```python
from build123d import *

# Parameters (mm, degrees)
F1_R     = 3.429
F2_DEPTH = 2.54
F3_DEPTH = 25.4


# Not quite as in the source:
# - a feature names something its author has since deleted; it is built from what else it names


with BuildPart() as f2:
    # F1 (on offset) → F2 (new body)
    with BuildSketch(Plane.XZ.offset(25.4)):
        with BuildLine():
            Line((-6.7237908952, -152.7482020624), (-6.7237908952, -156.4639806747))
            Line((-6.7237908952, -156.4639806747), (-2.04e-07, -156.4639806747))
            Line((-2.04e-07, -156.4639806747), (6.7237904873, -156.4639806747))
            Line((6.7237904873, -156.4639806747), (6.7237904873, -152.7482020624))
            Line((6.7237904873, -152.7482020624), (4.8364107652, -152.7482020624))
            Line((4.8364107652, -152.7482020624), (4.8364107652, -150.8608219091))
            Line((4.8364107652, -150.8608219091), (4.8364107652, -150.7428611076))
            Line((4.8364107652, -150.7428611076), (1.0616511053, -150.7428611076))
            Line((1.0616511053, -150.7428611076), (1.0616511053, 30.8865145628))
            ThreePointArc((1.0616511053, 30.8865145628), (-2.065e-07, 30.802726532), (-1.0616515132, 30.8865146276))
            Line((-1.0616515132, 30.8865146276), (-1.0616515132, -150.7428611076))
            Line((-1.0616515132, -150.7428611076), (-1.0616515132, -150.8608219091))
            Line((-1.0616515132, -150.8608219091), (-4.8364111731, -150.8608219091))
            Line((-4.8364111731, -150.8608219091), (-4.8364111731, -152.7482020624))
            Line((-4.8364111731, -152.7482020624), (-6.7237908952, -152.7482020624))
        make_face()
        with BuildLine():
            ThreePointArc((6.7678133299, 37.5705398619), (-4.3942142646, 42.7177894445), (-1.0616515132, 30.8865146276))
            ThreePointArc((-1.0616515132, 30.8865146276), (-2.065e-07, 30.802726532), (1.0616511053, 30.8865145628))
            ThreePointArc((1.0616511053, 30.8865145628), (5.1472494485, 33.1763254403), (6.7678133299, 37.5705398619))
        make_face()
        with Locations((0, 37.5705398619)):
            Circle(F1_R, mode=Mode.SUBTRACT)
        with Locations((0, 37.5705398619)):
            Circle(F1_R)
    extrude(amount=-F2_DEPTH)

    # F1 (on offset) → F3 (cut)
    with BuildSketch(Plane.XZ.offset(25.4)):
        with Locations((0, 37.5705398619)):
            Circle(F1_R)
    extrude(amount=-F3_DEPTH, mode=Mode.SUBTRACT)


solid = f2.part
```
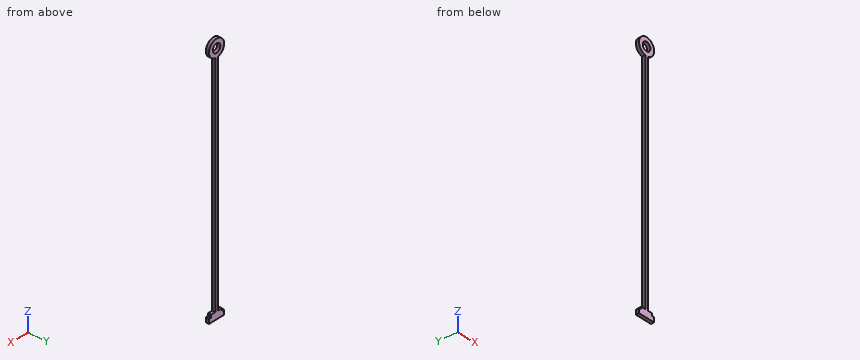
Geometry: final body of the model. Coordinates: model frame, mm. Coordinates: 2 decimals unless noted, no trailing zeros. Order: outer loops, then holes, each group sorted by start corner. A loop starts at its lowest first (then second) coordinate and runs counter-clockwise, first axis right, second up. Notation, with made-up numbers: M 41,-18.5 L 71,-18.5 A18 cw 71,8.5 Z; hole C -39,-22 d1. An arc over 180 degrees is marked long. Answer in a Markdown table with one row per item. Add a question column.
Q1. Line query: L1, parallel to Z at x = 0, y = -24.5; L2, parallel to X at y = -24.9, z = -57.5; L3, parallel to Z at x = 3.75, y = -25.15. Output: solid intervals per line, ascending.
Q2. Section query B-B on z = -62. Return the cut outline in (x, y).
Q3. Section query A-A on y = -23.55. Return the cut outline in (x, z).
Q4. Contact query for flat-ended pins moving along their axis: P1, Ø1.5, axis at x = 4, y = -24, coming from the +Z side; P2, Ø1.5, axis at y = -24, z = -134, coming from the +X side; P3, Ø1.5, axis at x = -6, y = -24.5, coming from the +Z side. Output: stop coordinate, or through.
Completed:
| question | item | result |
|---|---|---|
| 1 | L1 | z = -156.46 to 34.14, 41 to 44.34 |
| 1 | L2 | x = -1.06 to 1.06 |
| 1 | L3 | z = -156.46 to -150.74, 31.94 to 43.2 |
| 2 | outline | M -1.06,-25.4 L 1.06,-25.4 L 1.06,-22.86 L -1.06,-22.86 Z |
| 3 | outline | M -6.72,-156.46 L 6.72,-156.46 L 6.72,-152.75 L 4.84,-152.75 L 4.84,-150.74 L 1.06,-150.74 L 1.06,30.89 A6.77 ccw long -1.06,30.89 L -1.06,-150.86 L -4.84,-150.86 L -4.84,-152.75 L -6.72,-152.75 Z; hole C 0,37.57 d6.86 |
| 4 | P1 | stops at z = 43.51 |
| 4 | P2 | stops at x = 1.06 |
| 4 | P3 | stops at z = 41.84 |
